Design review of the part built by this model. Coordinates are the model's own, in mm. A direction names the side the tool comes from. Give positions to 0.01 mm unless a question says otherwise; leave off trailing zeros. Write each loop counter-clockwise with the first axis right and the second up, starting at its lowest first coordinate (ties: lowest second). Pieces come first, ordered by that corner, then holes.
```python
from build123d import *

# Parameters (mm, degrees)
SKETCH1_R                         = 190.5
BOSS_EXTRUDE1_DEPTH               = 50.8
SKETCH2_R                         = 63.5
CUT_EXTRUDE1_DEPTH                = 275.155320941
F_3_4_16_TAPPED_HOLE1_D           = 17.4625
F_3_4_16_TAPPED_HOLE1_DEPTH       = 42.926
F_3_4_16_TAPPED_HOLE1_CSINK_D     = 20.32
F_3_4_16_TAPPED_HOLE1_CSINK_ANGLE = 100
F_3_4_16_TAPPED_HOLE1_TIP         = 5.24626428
SKETCH5_R                         = 15.875
BOSS_EXTRUDE2_DEPTH               = 25.4


with BuildPart() as part:
    # Sketch1 → Boss-Extrude1 (new body)
    with BuildSketch(Plane.XY):
        Circle(SKETCH1_R)
    extrude(amount=BOSS_EXTRUDE1_DEPTH)

    # Sketch2 → Cut-Extrude1 (cut, through all)
    with BuildSketch(Plane.XY.offset(50.8)):
        Circle(SKETCH2_R)
    extrude(amount=-CUT_EXTRUDE1_DEPTH, mode=Mode.SUBTRACT)

    # 3/4-16 Tapped Hole1
    with Locations(Plane.XY.offset(50.8)):
        with Locations((0, 0), (0, 152.4), (0, 101.6), (71.842048969, 71.842048969), (101.6, 0), (107.763073453, 107.763073453), (71.842048969, -71.842048969), (0, -101.6), (-71.842048969, -71.842048969), (-101.6, 0), (-71.842048969, 71.842048969), (152.4, 0), (107.763073453, -107.763073453), (0, -152.4), (-107.763073453, -107.763073453), (-152.4, 0), (-107.763073453, 107.763073453)):
            CounterSinkHole(F_3_4_16_TAPPED_HOLE1_D / 2, F_3_4_16_TAPPED_HOLE1_CSINK_D / 2, depth=F_3_4_16_TAPPED_HOLE1_DEPTH, counter_sink_angle=F_3_4_16_TAPPED_HOLE1_CSINK_ANGLE)
            with Locations((0, 0, -(F_3_4_16_TAPPED_HOLE1_DEPTH + F_3_4_16_TAPPED_HOLE1_TIP / 2))):  # 118° drill point
                Cone(0, F_3_4_16_TAPPED_HOLE1_D / 2, F_3_4_16_TAPPED_HOLE1_TIP, mode=Mode.SUBTRACT)

    # Sketch5 → Boss-Extrude2 (add)
    with BuildSketch(Plane(origin=(0, 0, 0), x_dir=(-1, 0, 0), z_dir=(0, 0, -1))):
        with Locations(Location((0, 152.4, 0), (0, 0, 180))):
            Circle(SKETCH5_R)
        with Locations(Location((97.960831716, 116.745173131, 0), (0, 0, 180))):
            Circle(SKETCH5_R)
        with Locations(Location((150.084701559, 26.463982276, 0), (0, 0, 180))):
            Circle(SKETCH5_R)
        with Locations(Location((131.982271537, -76.2, 0), (0, 0, 180))):
            Circle(SKETCH5_R)
        with Locations(Location((52.123869843, -143.209155408, 0), (0, 0, 180))):
            Circle(SKETCH5_R)
        with Locations(Location((-52.123869843, -143.209155408, 0), (0, 0, 180))):
            Circle(SKETCH5_R)
        with Locations(Location((-131.982271537, -76.2, 0), (0, 0, 180))):
            Circle(SKETCH5_R)
        with Locations(Location((-150.084701559, 26.463982276, 0), (0, 0, 180))):
            Circle(SKETCH5_R)
        with Locations(Location((-97.960831716, 116.745173131, 0), (0, 0, 180))):
            Circle(SKETCH5_R)
    extrude(amount=BOSS_EXTRUDE2_DEPTH)


solid = part.part
```
(1) Consider section C-C, the plane x = 128. Give the boundary of the cut face in (y, z).
Resolved:
outline: (-141.09, 0) - (-91.57, 0) - (-91.57, -25.4) - (-60.83, -25.4) - (-60.83, 0) - (141.09, 0) - (141.09, 50.8) - (-141.09, 50.8) - close
(2) Tool access review of faces 4 (the face through (-13.77, -61.99, 25.76)), 5 (the face through (-63.12, -71.46, 28.45)), 6 (the face through (-165.944, 25.766, -12.522)): name each direction out of +Z, -Z, +X, -X, +Y, -Y from which nothing blocks a thin tool from reaching the whole face with its end or side.
Resolved:
face 4: +Z, -Z
face 5: +Z
face 6: -Z
(3) Clearance check with flat-ended pins moving along their axes: P1, Ø4, axis at y = -83.5, z = 15.5, coming from the -X side; P2, Ø14, axis at x = 0, y = 152.4, coming from the +Z side; P3, Ø15.5, axis at x = 0, y = -101.6, coming from the +Z side. State where each tip first meets the part, or that it passes through.
Resolved:
P1: stops at x = -172.19
P2: stops at z = 6.83
P3: stops at z = 7.28
(4) Consider section B-B, the plane z = -12. Give the number of separate pieces and of enclosed holes in the cut face, then the cut area to 3 significant figures.
Resolved:
separate pieces: 9
enclosed holes: 0
area: 7,130 mm2
(5) Mouldability with a two-part tool opening along X and no side actions: class faces 1 (the face through (80.565, -71.458, 28.445)), 2 (the face through (150, 26, -25.4)), 3 (the face through (7.33, 166.48, -12.52)) as pulls with the +X half, pulls with the -X half, needs draft (parallel to the pull), parting line crosses it, or undercut.
Resolved:
face 1: undercut
face 2: needs draft
face 3: parting line crosses it
(6) Consider section A-A, the plane y = 53. Give the boundary of the cut face in (x, z) (3 decimals).
Resolved:
outline: (-182.979, 0) - (-34.975, 0) - (-34.975, 50.8) - (-182.979, 50.8) - close; (34.975, 0) - (182.979, 0) - (182.979, 50.8) - (34.975, 50.8) - close
(7) To check wall thickness, follow L1, parallel to X at y = -101.6, z = 23; L2, parallel to X at y = 116, z = -4; L3, parallel to Y at x = 101, z = 16. State the ranges of each line that lie inside material, in increasing order.
Resolved:
L1: x = -161.14 to -113.95, -101.58 to -8.73, 8.73 to 101.58, 113.95 to 161.14
L2: x = -113.82 to -82.1, 82.1 to 113.82
L3: y = -161.52 to -113.29, -102.24 to -8.71, 8.71 to 102.24, 113.29 to 161.52
